from build123d import *

# Parameters (mm, degrees)
BOSS_EXTRUDE1_DEPTH     = 10
SKETCH2_W               = 5
SKETCH2_H               = 4
CUT_EXTRUDE1_DEPTH      = 79
BOSS_EXTRUDE2_DEPTH     = 13
CUT_EXTRUDE2_DEPTH      = 100.097174531
CUT_EXTRUDE2_DEPTH_BACK = 100.097174531
SKETCH6_W               = 5
SKETCH6_H               = 65
SKETCH7_R               = 6
CUT_EXTRUDE3_DEPTH      = 13
RIB1_REACH              = 93.707
SKETCH8_WALL_W          = 231.065679212
SKETCH8_WALL_H          = 10
SKETCH9_R               = 6
CUT_EXTRUDE4_DEPTH      = 13


with BuildPart() as part:
    # Sketch1 → Boss-Extrude1 (new body)
    with BuildSketch(Plane(origin=(0, 0, 0), x_dir=(1, 0, 0), z_dir=(0, 1, 0))):
        with BuildLine():
            Line((-39.5, 0), (39.5, 0))
            Line((39.5, 0), (39.5, -23))
            ThreePointArc((39.5, -23), (35.985281374, -31.485281374), (27.5, -35))
            Line((27.5, -35), (-27.5, -35))
            ThreePointArc((-27.5, -35), (-35.985281374, -31.485281374), (-39.5, -23))
            Line((-39.5, -23), (-39.5, 0))
        make_face()
    extrude(amount=BOSS_EXTRUDE1_DEPTH)

    # Sketch2 → Cut-Extrude1 (cut)
    with BuildSketch(Plane(origin=(39.5, 0, 0), x_dir=(0, 0, -1), z_dir=(1, 0, 0))):
        with Locations((-2.5, 8)):
            Rectangle(SKETCH2_W, SKETCH2_H)
    extrude(amount=-CUT_EXTRUDE1_DEPTH, mode=Mode.SUBTRACT)

    # Sketch5 → Boss-Extrude2 (add)
    with BuildSketch(Plane.XY):
        with BuildLine():
            Line((-15, 60), (-15, 21.608186766))
            ThreePointArc((-15, 21.608186766), (-16.444558288, 15.185570477), (-20.5, 10))
            Line((-20.5, 10), (20.5, 10))
            ThreePointArc((20.5, 10), (16.444558288, 15.185570477), (15, 21.608186766))
            Line((15, 21.608186766), (15, 60))
            ThreePointArc((15, 60), (0, 75), (-15, 60))
        make_face()
    extrude(amount=BOSS_EXTRUDE2_DEPTH)

    # Sketch6 → Cut-Extrude2 (cut, two sides: drawn at the far end of the back side and taken through both)
    with BuildSketch(Plane(origin=(15, 0, 0), x_dir=(0, 0, -1), z_dir=(1, 0, 0)).offset(-CUT_EXTRUDE2_DEPTH_BACK)):
        with Locations((-2.5, 42.5)):
            Rectangle(SKETCH6_W, SKETCH6_H)
    extrude(amount=CUT_EXTRUDE2_DEPTH + CUT_EXTRUDE2_DEPTH_BACK, mode=Mode.SUBTRACT)

    # Sketch7 → Cut-Extrude3 (cut)
    with BuildSketch(Plane.XY.offset(13)):
        with Locations((0, 60)):
            Circle(SKETCH7_R)
    extrude(amount=-CUT_EXTRUDE3_DEPTH, mode=Mode.SUBTRACT)

    # Sketch8 wall → Rib1 (add, up to next)
    with BuildSketch(Plane(origin=(0, 30, 24), x_dir=(0, 0.876215908677, -0.481918749772), z_dir=(0, 0.481918749772, 0.876215908677)), mode=Mode.PRIVATE) as rib1_sk1:
        Rectangle(SKETCH8_WALL_W, SKETCH8_WALL_H)
    rib1_tool1 = extrude(rib1_sk1.sketch, amount=-RIB1_REACH, mode=Mode.PRIVATE) - part.part
    add(rib1_tool1.solids().sort_by_distance((0, 30, 24))[0])

    # Sketch9 → Cut-Extrude4 (cut)
    with BuildSketch(Plane(origin=(0, 10, 0), x_dir=(1, 0, 0), z_dir=(0, 1, 0))):
        with Locations(Location((23, -20, 0), (0, 0, 270))):
            Circle(SKETCH9_R)
        with Locations(Location((-23, -20, 0), (0, 0, 270))):
            Circle(SKETCH9_R)
    extrude(amount=-CUT_EXTRUDE4_DEPTH, mode=Mode.SUBTRACT)


solid = part.part
The model under review builds one solid part; all positions refer to its coordinate system, in mm. A direction names the side the tool comes from. Round coordinates to 2 decimals unless told otherwise and drop trailing zeros. Write each loop counter-clockwise with the first axis right and the second up, starting at its lowest first coordinate (ties: lowest second). Pieces come first, ordered by that corner, then holes. Notation, with made-up numbers: M 50,89 L 59,89 A23 ccw 59,110 Z; hole C -37,19 d1. An arc over 180 degrees is marked long. Use a Markdown table: item, result. Add a question column.
Q1. Machinability: for faces 4 (the face through (22.5, 10, 26.5)), 5 (the face through (-22, 10, 26.5)), 6 (the face through (-1, 32, 5)), 7 (the face through (15, 41, 9)), which of the approach directions +Z, -Z, +X, -X, +Y, -Y give a long, thin tool a straight path to every point of the face, cutting with its end or side? Answer none if there is none.
Q2. To check wall thickness, follow line 1 (X direction, y = 6, z = 20); line 2 (X direction, y = 4, z = 25); line 3 (Y direction, x = 0, z = 9.25). State the ranges of each line that lie inside material, in increasing order.
Q3. Insertion check: pin 1 (15 mm diameter, centred on x = 14, z = 27.5, fed in from +Y); pin 2 (6.5 mm diameter, centred on y = 49.5, z = 10.5, fed in from -X); pin 3 (6 mm diameter, centred on x = -15.5, y = 38.5, fed in from +Z); pin 4 (11 mm diameter, centred on x = -23, z = 20, fed in from -Y). Each pin has a flat end and moves straight along its axis. Give the tip position at first contact, or say it passes through.
Q4. We need section A-A, the plane x = 0. State the section outline as (y, z) points.
Q5. We need section B-B, the plane z = 6.5. State the section outline as (x, y) points.
Q6. We need section C-C, the plane y = 25. State the section outline as (x, z) points.
Q7. We need section D-D, the plane z = 18.5. State the section outline as (x, y) points.
Q8. The part is to be moulded in two halves that separate along X. For faces 1 (the face through (-16.405, 15.27, 8.944)), 2 (the face through (-1, 3, 0)), 3 (the face through (-25.3, 5.07, 25.54)), say which applies: pulls with the +X half, pulls with the -X half, needs draft (parallel to the pull), parting line crosses it, or undercut.
Findings below:
| question | item | result |
|---|---|---|
| 1 | face 4 | +Z, +X, +Y |
| 1 | face 5 | +Z, -X, +Y |
| 1 | face 6 | -Z, +X, -X, +Y |
| 1 | face 7 | +Z, -Z, +X, +Y |
| 2 | line 1 | x = -39.5 to -29, -17 to 17, 29 to 39.5 |
| 2 | line 2 | x = -39.33 to -26.32, -19.68 to 19.68, 26.32 to 39.33 |
| 2 | line 3 | y = 0 to 54, 66 to 75 |
| 3 | pin 1 | stops at y = 10 |
| 3 | pin 2 | stops at x = -15 |
| 3 | pin 3 | stops at z = 13 |
| 3 | pin 4 | passes through |
| 4 | outline | M 0,0 L 6,0 L 6,5 L 54,5 L 54,13 L 50,13 L 10,35 L 0,35 Z; M 66,5 L 75,5 L 75,13 L 66,13 Z |
| 5 | outline | M -39.5,0 L 39.5,0 L 39.5,10 L 20.5,10 A15 cw 15,21.61 L 15,60 A15 ccw -15,60 L -15,21.61 A15 cw -20.5,10 L -39.5,10 Z; hole C 0,60 d12 |
| 6 | outline | M -15,5 L 15,5 L 15,13 L 5,13 L 5,26.75 L -5,26.75 L -5,13 L -15,13 Z |
| 7 | outline | M -39.5,0 L -28.81,0 L -28.81,10 L -39.5,10 Z; M -17.19,0 L 17.19,0 L 17.19,10 L 5,10 L 5,40 L -5,40 L -5,10 L -17.19,10 Z; M 28.81,0 L 39.5,0 L 39.5,10 L 28.81,10 Z |
| 8 | face 1 | pulls with the -X half |
| 8 | face 2 | needs draft |
| 8 | face 3 | undercut |
